Geometry: final body of the model. Coordinates: model frame, mm. A direction names the side the tool comes from. Give positions to 0.01 mm unless a question says otherwise; leave off trailing zeros. Loops run counter-clockwise (first coordinate to the right, second up) from the corner with the lowest first, then second, coordinate; pieces in that order, holes last.
from build123d import *

# Parameters (mm, degrees)
BOX114_W          = 9
BOX114_H          = 1
BOX114_DEPTH      = 1
CYLINDER025_R     = 0.5
CYLINDER025_DEPTH = 3
CYLINDER023_R     = 0.5
CYLINDER023_DEPTH = 3
CYLINDER024_R     = 0.5
CYLINDER024_DEPTH = 3
CYLINDER026_R     = 0.5
CYLINDER026_DEPTH = 3
CYLINDER021_R     = 0.5
CYLINDER021_DEPTH = 3
CYLINDER020_R     = 0.5
CYLINDER020_DEPTH = 3
CYLINDER019_R     = 0.5
CYLINDER019_DEPTH = 3
CYLINDER022_R     = 0.5
CYLINDER022_DEPTH = 3
BOX113_W          = 9
BOX113_H          = 1
BOX113_DEPTH      = 1
CYLINDER007_R     = 0.5
CYLINDER007_DEPTH = 3
CYLINDER009_R     = 0.5
CYLINDER009_DEPTH = 3
CYLINDER008_R     = 0.5
CYLINDER008_DEPTH = 3
CYLINDER010_R     = 0.5
CYLINDER010_DEPTH = 3
CYLINDER011_R     = 0.5
CYLINDER011_DEPTH = 3
CYLINDER013_R     = 0.5
CYLINDER013_DEPTH = 3
CYLINDER012_R     = 0.5
CYLINDER012_DEPTH = 3
CYLINDER014_R     = 0.5
CYLINDER014_DEPTH = 3
CYLINDER015_R     = 0.5
CYLINDER015_DEPTH = 3
CYLINDER016_R     = 0.5
CYLINDER016_DEPTH = 3
CYLINDER017_R     = 0.5
CYLINDER017_DEPTH = 3
CYLINDER018_R     = 0.5
CYLINDER018_DEPTH = 3
CYLINDER006_R     = 0.5
CYLINDER006_DEPTH = 3
BOX112_W          = 1
BOX112_H          = 25
BOX112_DEPTH      = 1
BOX115_W          = 1
BOX115_H          = 6
BOX115_DEPTH      = 1
BOX116_W          = 1
BOX116_H          = 6
BOX116_DEPTH      = 1


with BuildPart() as box114:
    # Box114 → Box114 (new body)
    with BuildSketch(Plane(origin=(-9, 24, 14), x_dir=(1, 0, 0), z_dir=(0, 0, 1))):
        with Locations((4.5, 0.5)):
            Rectangle(BOX114_W, BOX114_H)
    extrude(amount=BOX114_DEPTH)


with BuildPart() as cylinder025:
    # Cylinder025 → Cylinder025 (new body)
    with BuildSketch(Plane(origin=(-1.5, 0.5, 11), x_dir=(1, 0, 0), z_dir=(0, 0, 1))):
        Circle(CYLINDER025_R)
    extrude(amount=CYLINDER025_DEPTH)


with BuildPart() as cylinder023:
    # Cylinder023 → Cylinder023 (new body)
    with BuildSketch(Plane(origin=(-7.5, 0.5, 11), x_dir=(1, 0, 0), z_dir=(0, 0, 1))):
        Circle(CYLINDER023_R)
    extrude(amount=CYLINDER023_DEPTH)


with BuildPart() as cylinder024:
    # Cylinder024 → Cylinder024 (new body)
    with BuildSketch(Plane(origin=(-5.5, 0.5, 11), x_dir=(1, 0, 0), z_dir=(0, 0, 1))):
        Circle(CYLINDER024_R)
    extrude(amount=CYLINDER024_DEPTH)


with BuildPart() as fusion057:
    # Cylinder026 → Cylinder026 (new body)
    with BuildSketch(Plane(origin=(-3.5, 0.5, 11), x_dir=(1, 0, 0), z_dir=(0, 0, 1))):
        Circle(CYLINDER026_R)
    extrude(amount=CYLINDER026_DEPTH)

    # Fusion056: union Cylinder025, Cylinder023, Cylinder024
    add(cylinder025.part)
    add(cylinder023.part)
    add(cylinder024.part)


with BuildPart() as fusion057_1:
    # Fusion056 placement: moved
    add(fusion057.part.moved(Location((0, 24, 0))))

    # Fusion057: union Box114
    add(box114.part)


with BuildPart() as cylinder021:
    # Cylinder021 → Cylinder021 (new body)
    with BuildSketch(Plane(origin=(-1.5, 0.5, 11), x_dir=(1, 0, 0), z_dir=(0, 0, 1))):
        Circle(CYLINDER021_R)
    extrude(amount=CYLINDER021_DEPTH)


with BuildPart() as cylinder020:
    # Cylinder020 → Cylinder020 (new body)
    with BuildSketch(Plane(origin=(-7.5, 0.5, 11), x_dir=(1, 0, 0), z_dir=(0, 0, 1))):
        Circle(CYLINDER020_R)
    extrude(amount=CYLINDER020_DEPTH)


with BuildPart() as cylinder019:
    # Cylinder019 → Cylinder019 (new body)
    with BuildSketch(Plane(origin=(-5.5, 0.5, 11), x_dir=(1, 0, 0), z_dir=(0, 0, 1))):
        Circle(CYLINDER019_R)
    extrude(amount=CYLINDER019_DEPTH)


with BuildPart() as fusion055:
    # Cylinder022 → Cylinder022 (new body)
    with BuildSketch(Plane(origin=(-3.5, 0.5, 11), x_dir=(1, 0, 0), z_dir=(0, 0, 1))):
        Circle(CYLINDER022_R)
    extrude(amount=CYLINDER022_DEPTH)

    # Fusion055: union Cylinder021, Cylinder020, Cylinder019
    add(cylinder021.part)
    add(cylinder020.part)
    add(cylinder019.part)


with BuildPart() as fusion058:
    # Box113 → Box113 (new body)
    with BuildSketch(Plane(origin=(-9, 0, 14), x_dir=(1, 0, 0), z_dir=(0, 0, 1))):
        with Locations((4.5, 0.5)):
            Rectangle(BOX113_W, BOX113_H)
    extrude(amount=BOX113_DEPTH)

    # Fusion058: union Fusion055
    add(fusion055.part)


with BuildPart() as cylinder007:
    # Cylinder007 → Cylinder007 (new body)
    with BuildSketch(Plane(origin=(-9.5, 2.5, 11), x_dir=(1, 0, 0), z_dir=(0, 0, 1))):
        Circle(CYLINDER007_R)
    extrude(amount=CYLINDER007_DEPTH)


with BuildPart() as cylinder009:
    # Cylinder009 → Cylinder009 (new body)
    with BuildSketch(Plane(origin=(-9.5, 6.5, 11), x_dir=(1, 0, 0), z_dir=(0, 0, 1))):
        Circle(CYLINDER009_R)
    extrude(amount=CYLINDER009_DEPTH)


with BuildPart() as cylinder008:
    # Cylinder008 → Cylinder008 (new body)
    with BuildSketch(Plane(origin=(-9.5, 4.5, 11), x_dir=(1, 0, 0), z_dir=(0, 0, 1))):
        Circle(CYLINDER008_R)
    extrude(amount=CYLINDER008_DEPTH)


with BuildPart() as cylinder010:
    # Cylinder010 → Cylinder010 (new body)
    with BuildSketch(Plane(origin=(-9.5, 8.5, 11), x_dir=(1, 0, 0), z_dir=(0, 0, 1))):
        Circle(CYLINDER010_R)
    extrude(amount=CYLINDER010_DEPTH)


with BuildPart() as cylinder011:
    # Cylinder011 → Cylinder011 (new body)
    with BuildSketch(Plane(origin=(-9.5, 10.5, 11), x_dir=(1, 0, 0), z_dir=(0, 0, 1))):
        Circle(CYLINDER011_R)
    extrude(amount=CYLINDER011_DEPTH)


with BuildPart() as cylinder013:
    # Cylinder013 → Cylinder013 (new body)
    with BuildSketch(Plane(origin=(-9.5, 14.5, 11), x_dir=(1, 0, 0), z_dir=(0, 0, 1))):
        Circle(CYLINDER013_R)
    extrude(amount=CYLINDER013_DEPTH)


with BuildPart() as cylinder012:
    # Cylinder012 → Cylinder012 (new body)
    with BuildSketch(Plane(origin=(-9.5, 12.5, 11), x_dir=(1, 0, 0), z_dir=(0, 0, 1))):
        Circle(CYLINDER012_R)
    extrude(amount=CYLINDER012_DEPTH)


with BuildPart() as cylinder014:
    # Cylinder014 → Cylinder014 (new body)
    with BuildSketch(Plane(origin=(-9.5, 16.5, 11), x_dir=(1, 0, 0), z_dir=(0, 0, 1))):
        Circle(CYLINDER014_R)
    extrude(amount=CYLINDER014_DEPTH)


with BuildPart() as cylinder015:
    # Cylinder015 → Cylinder015 (new body)
    with BuildSketch(Plane(origin=(-9.5, 18.5, 11), x_dir=(1, 0, 0), z_dir=(0, 0, 1))):
        Circle(CYLINDER015_R)
    extrude(amount=CYLINDER015_DEPTH)


with BuildPart() as cylinder016:
    # Cylinder016 → Cylinder016 (new body)
    with BuildSketch(Plane(origin=(-9.5, 20.5, 11), x_dir=(1, 0, 0), z_dir=(0, 0, 1))):
        Circle(CYLINDER016_R)
    extrude(amount=CYLINDER016_DEPTH)


with BuildPart() as cylinder017:
    # Cylinder017 → Cylinder017 (new body)
    with BuildSketch(Plane(origin=(-9.5, 22.5, 11), x_dir=(1, 0, 0), z_dir=(0, 0, 1))):
        Circle(CYLINDER017_R)
    extrude(amount=CYLINDER017_DEPTH)


with BuildPart() as cylinder018:
    # Cylinder018 → Cylinder018 (new body)
    with BuildSketch(Plane(origin=(-9.5, 24.5, 11), x_dir=(1, 0, 0), z_dir=(0, 0, 1))):
        Circle(CYLINDER018_R)
    extrude(amount=CYLINDER018_DEPTH)


with BuildPart() as fusion053:
    # Cylinder006 → Cylinder006 (new body)
    with BuildSketch(Plane(origin=(-9.5, 0.5, 11), x_dir=(1, 0, 0), z_dir=(0, 0, 1))):
        Circle(CYLINDER006_R)
    extrude(amount=CYLINDER006_DEPTH)

    # Fusion053: union Cylinder007, Cylinder009, Cylinder008, Cylinder010, Cylinder011, Cylinder013, Cylinder012, Cylinder014, Cylinder015, Cylinder016, Cylinder017, Cylinder018
    add(cylinder007.part)
    add(cylinder009.part)
    add(cylinder008.part)
    add(cylinder010.part)
    add(cylinder011.part)
    add(cylinder013.part)
    add(cylinder012.part)
    add(cylinder014.part)
    add(cylinder015.part)
    add(cylinder016.part)
    add(cylinder017.part)
    add(cylinder018.part)


with BuildPart() as fusion060:
    # Box112 → Box112 (new body)
    with BuildSketch(Plane(origin=(-10, 0, 14), x_dir=(1, 0, 0), z_dir=(0, 0, 1))):
        with Locations((0.5, 12.5)):
            Rectangle(BOX112_W, BOX112_H)
    extrude(amount=BOX112_DEPTH)

    # Fusion054: union Fusion053
    add(fusion053.part)

    # Fusion060: union Fusion057, Fusion058
    add(fusion057_1.part)
    add(fusion058.part)


with BuildPart() as box115:
    # Box115 → Box115 (new body)
    with BuildSketch(Plane.XY.offset(14)):
        with Locations((0.5, 3)):
            Rectangle(BOX115_W, BOX115_H)
    extrude(amount=BOX115_DEPTH)


with BuildPart() as fusion062:
    # Box116 → Box116 (new body)
    with BuildSketch(Plane(origin=(0, 19, 14), x_dir=(1, 0, 0), z_dir=(0, 0, 1))):
        with Locations((0.5, 3)):
            Rectangle(BOX116_W, BOX116_H)
    extrude(amount=BOX116_DEPTH)

    # Fusion061: union Box115
    add(box115.part)

    # Fusion062: union Fusion060
    add(fusion060.part)


solid = fusion062.part
Item 1: Set-up query: faces 3 (the face through (0, 3.5, 14.5)), 4 (the face through (0.5, 19, 14.5)), 5 (the face through (-5.565, 24.996, 12.479)). Return all of +Z, -Z, +X, -X, +Y, -Y with unobstructed straight access to the full face (end or side cutting, diameter ignored); none if empty.
Values follow:
face 3: +Z, -Z
face 4: +Z, -Z, +X
face 5: -Z
Item 2: Ray query, probe 1 along Y at (x, z) = (-6.5, 14.8); probe 2 along Z at (x, y) = (0.25, 23.25); probe 3 along X at (y, z) = (14.5, 12.8). Return the intervals inside material, ascending.
Values follow:
probe 1: y = 0 to 1, 24 to 25
probe 2: z = 14 to 15
probe 3: x = -10 to -9
Item 3: Section query D-D on y = 13.25. Return loops of the section in (x, z).
Values follow:
outline: (-10, 14) - (-9, 14) - (-9, 15) - (-10, 15) - close
Item 4: Draft query along Y for faces 1 (the face through (-9.5, 6.5, 11)), 2 (the face through (-5.9, 0.2, 12.5)). Return one class per face: +Y half, -Y half, draft (parallel to the pull), parting line (faces both ways), or undercut.
Values follow:
face 1: draft
face 2: undercut
Item 5: Section query A-A on x = -0.75. Return loops of the section in (y, z), plus the area to 3 significant figures.
Values follow:
outline: (0, 14) - (1, 14) - (1, 15) - (0, 15) - close; (24, 14) - (25, 14) - (25, 15) - (24, 15) - close
area: 2.00 mm2
Item 6: Section query B-B on z = 13.4. Give the number of separate pieces and of enclosed holes in the cut face, plus the area to 3 significant figures.
Values follow:
separate pieces: 21
enclosed holes: 0
area: 16.5 mm2
Item 7: Pin query (flat end, axial travel): pin 1 (0.5 mm diameter, centred on x = -2.5, y = 24.5, fed in from -Z); pin 2 (6 mm diameter, centred on x = -5, y = 8.5, fed in from +Z). Return the tip coordinate at first contact, or that it passes through.
Values follow:
pin 1: stops at z = 14
pin 2: passes through
Item 8: Section query C-C on z = 14.6. Return loops of the section in (x, y).
Values follow:
outline: (-10, 0) - (1, 0) - (1, 6) - (0, 6) - (0, 1) - (-9, 1) - (-9, 24) - (0, 24) - (0, 19) - (1, 19) - (1, 25) - (-10, 25) - close
